Read the model definition and answer for the solid it produces. Units are mm, in the model's axes. Coordinates: 2 decimals unless noted, no trailing zeros. Write each loop counter-clockwise with the first axis right and the second up, starting at its lowest first coordinate (ties: lowest second). Pieces come first, ordered by that corner, then holes.
Item 1: Section A-A (z = 203.2) is taken. Give the vertices of the cut face in (x, y), then the cut area to 3 significant figures.
Item 2: Section D-D (x = 90.5) is taken. State how many separate pieces and enclosed holes the cut face has, then the cut area to 3 significant figures.
Item 3: Straight lines are drawn through the part: probe 1 along Z at (x, y) = (93.75, -31.75); probe 2 along Y at (x, z) = (92.5, 190.5); probe 3 along Z at (x, y) = (94, -95.25). For each, find the intervals that lie inside material, in ascending order.
Item 4: This flat-tipped pin is pushed along its axis until it touches: P1, Ø2, axis at x = 90, z = 188.5, coming from the -Y side. Where does it stop, or does it pass through?
Item 5: Determine the mould class of faces 1 (the face through (92.12, -20.86, 220.34)), 2 (the face through (92.12, -112.39, 220.44)), 3 (the face through (92.119, -83.883, 191.305)) for opening direction Y: released by +Y, released by -Y, zero draft, split by the parting line, or undercut.
Item 6: Section B-B (y = -31.75) is taken. Give the vertices of the cut face in (x, z), then the cut area to 3 significant figures.
Item 7: Section C-C (y = -93.5) is taken. Give the vertices of the cut face in (x, z).
from build123d import *

# Parameters (mm, degrees)
SKETCH1_R           = 1.7272
SKETCH1_R_2         = 14.2875
SKETCH1_R_3         = 2.4892
BOSS_EXTRUDE1_DEPTH = 6.35


with BuildPart() as part:
    # Sketch1 → Boss-Extrude1 (new body)
    with BuildSketch(Plane(origin=(95.25, 0, 0), x_dir=(0, 0, -1), z_dir=(1, 0, 0))):
        with BuildLine():
            Line((-184.15, -107.95), (-184.15, -25.4))
            ThreePointArc((-184.15, -25.4), (-186.009871939, -20.909871939), (-190.5, -19.05))
            Line((-190.5, -19.05), (-215.9, -19.05))
            ThreePointArc((-215.9, -19.05), (-220.390128061, -20.909871939), (-222.25, -25.4))
            Line((-222.25, -25.4), (-222.25, -107.95))
            ThreePointArc((-222.25, -107.95), (-220.390128061, -112.440128061), (-215.9, -114.3))
            Line((-215.9, -114.3), (-190.5, -114.3))
            ThreePointArc((-190.5, -114.3), (-186.009871939, -112.440128061), (-184.15, -107.95))
        make_face()
        with Locations(Location((-190.376194259, -82.426194259, 0), (0, 0, 180))):
            Circle(SKETCH1_R, mode=Mode.SUBTRACT)
        with Locations(Location((-216.023805741, -108.073805741, 0), (0, 0, 180))):
            Circle(SKETCH1_R, mode=Mode.SUBTRACT)
        with Locations(Location((-203.2, -95.25, 0), (0, 0, 180))):
            Circle(SKETCH1_R_2, mode=Mode.SUBTRACT)
        with Locations(Location((-215.9, -31.75, 0), (0, 0, 180))):
            Circle(SKETCH1_R_3, mode=Mode.SUBTRACT)
        with Locations(Location((-190.5, -31.75, 0), (0, 0, 180))):
            Circle(SKETCH1_R_3, mode=Mode.SUBTRACT)
        with Locations(Location((-215.9, -57.15, 0), (0, 0, 180))):
            Circle(SKETCH1_R_3, mode=Mode.SUBTRACT)
        with Locations(Location((-190.5, -57.15, 0), (0, 0, 180))):
            Circle(SKETCH1_R_3, mode=Mode.SUBTRACT)
    extrude(amount=-BOSS_EXTRUDE1_DEPTH)


solid = part.part
Established:
1. outline: (88.9, -114.3) - (95.25, -114.3) - (95.25, -109.54) - (88.9, -109.54) - close; (88.9, -80.96) - (95.25, -80.96) - (95.25, -19.05) - (88.9, -19.05) - close
1. area: 423 mm2
2. separate pieces: 1
2. enclosed holes: 7
2. area: 2,860 mm2
3. probe 1: z = 184.15 to 188.01, 192.99 to 213.41, 218.39 to 222.25
3. probe 2: y = -114.3 to -101.8, -88.7 to -84.15, -80.7 to -59.64, -54.66 to -34.24, -29.26 to -19.05
3. probe 3: z = 184.15 to 188.91, 217.49 to 222.25
4. P1: stops at y = -114.22
5. face 1: released by +Y
5. face 2: released by -Y
5. face 3: undercut
6. outline: (88.9, 184.15) - (95.25, 184.15) - (95.25, 188.01) - (88.9, 188.01) - close; (88.9, 192.99) - (95.25, 192.99) - (95.25, 213.41) - (88.9, 213.41) - close; (88.9, 218.39) - (95.25, 218.39) - (95.25, 222.25) - (88.9, 222.25) - close
6. area: 179 mm2
7. outline: (88.9, 184.15) - (95.25, 184.15) - (95.25, 189.02) - (88.9, 189.02) - close; (88.9, 217.38) - (95.25, 217.38) - (95.25, 222.25) - (88.9, 222.25) - close
